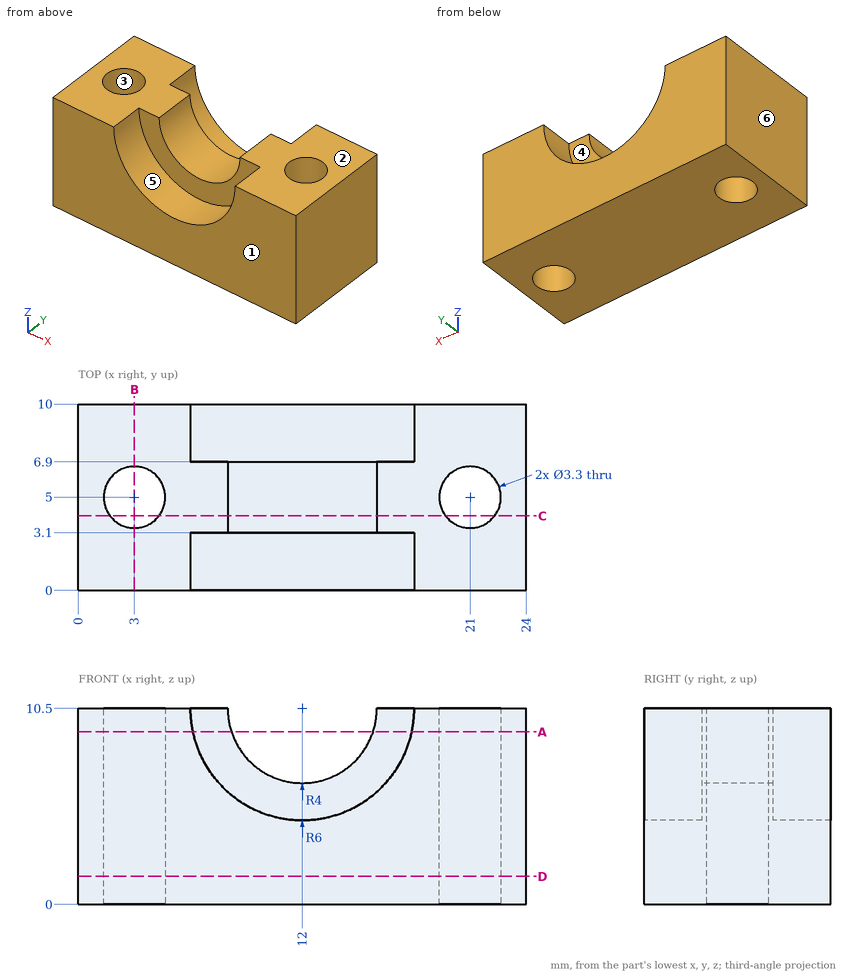
Geometry: see drawing. Coordinates: mm, zero at the bounding-box minimum. A direction names the side the tool comes from. Coordinates: 2 decimals unless noted, no trailing zeros. Loops run counter-clockwise (first coordinate to the right, second up) from the corner with the lowest first, then second, coordinate; pieces in that order, holes last. Notation, with made-up numbers: (24, 8.5) -> (62, 8.5) arc R24 ccw to (62, 28.5) -> close; hole circle Ø11 at (-21, 7). An arc over 180 degrees is marked (long way). Use a Markdown table: item, result.
1) Cut plane D-D (z = 1.5). Return the cut outline in (x, y).
Results found:
| item | result |
|---|---|
| outline | (0, 0) -> (24, 0) -> (24, 10) -> (0, 10) -> close; hole circle Ø3.3 at (3, 5); hole circle Ø3.3 at (21, 5) |
2) Access query for the marked faces 4, 5 and 6. Directions: +Z, -Z, +X, -X, +Y, -Y. A direction counts if a zero-diameter tool reaches every point of the face in a straight line with its end or side. Return the directions, or none.
Results found:
| item | result |
|---|---|
| face 4 | +Z, +Y |
| face 5 | +Z, -Y |
| face 6 | +Z, -Z, -X, +Y, -Y |
3) Cut plane C-C (y = 4). Return the cut outline in (x, z), then the cut area to 3 significant figures.
Results found:
| item | result |
|---|---|
| outline | (0, 0) -> (1.69, 0) -> (1.69, 10.5) -> (0, 10.5) -> close; (4.31, 0) -> (19.69, 0) -> (19.69, 10.5) -> (16, 10.5) arc R4 cw to (8, 10.5) -> (4.31, 10.5) -> close; (22.31, 0) -> (24, 0) -> (24, 10.5) -> (22.31, 10.5) -> close |
| area | 172 mm2 |
4) Material intervals for line 1 along Y through (x, z) = (21, 4); line 2 along X through (y, z) = (3.5, 3.5); line 3 along X through (y, z) = (2, 10.25), sorted ascending. Write a range as from..to.
Results found:
| item | result |
|---|---|
| line 1 | y = 0..3.35, 6.65..10 |
| line 2 | x = 0..2.31, 3.69..20.31, 21.69..24 |
| line 3 | x = 0..6.01, 17.99..24 |
5) Cut plane B-B (x = 3). Return the cut outline in (y, z), then the cut area to 4 significant figures.
Results found:
| item | result |
|---|---|
| outline | (0, 0) -> (3.35, 0) -> (3.35, 10.5) -> (0, 10.5) -> close; (6.65, 0) -> (10, 0) -> (10, 10.5) -> (6.65, 10.5) -> close |
| area | 70.35 mm2 |
6) Pull-direction query (Y, two-part tool) for the marked faces 1, 2 and 3; classes: released by +Y, released by -Y, zero draft, split by the parting line, or undercut.
Results found:
| item | result |
|---|---|
| face 1 | released by -Y |
| face 2 | zero draft |
| face 3 | undercut |
7) Contact query for flat-ended pins moving along their axis: pin 1 (3 mm diameter, centred on x = 15, z = 8, fed in from +Y); pin 2 (5 mm diameter, centred on x = 13, y = 6, fed in from +Z); pin 3 (3 mm diameter, centred on x = 12.5, z = 9, fed in from -Y). Output: stop coordinate, or through.
Results found:
| item | result |
|---|---|
| pin 1 | stops at y = 6.9 |
| pin 2 | stops at z = 8.56 |
| pin 3 | passes through |
8) Cut plane A-A (z = 9.25). Return the cut outline in (x, y), then the cut area to 3 significant figures.
Results found:
| item | result |
|---|---|
| outline | (0, 0) -> (6.13, 0) -> (6.13, 3.1) -> (8.2, 3.1) -> (8.2, 6.9) -> (6.13, 6.9) -> (6.13, 10) -> (0, 10) -> close; (15.8, 3.1) -> (17.87, 3.1) -> (17.87, 0) -> (24, 0) -> (24, 10) -> (17.87, 10) -> (17.87, 6.9) -> (15.8, 6.9) -> close; hole circle Ø3.3 at (3, 5); hole circle Ø3.3 at (21, 5) |
| area | 121 mm2 |
